Work out the finished part from the listing and answer in its coordinate system (mm). A direction names the side the tool comes from. Give positions to 0.01 mm unless a question says otherwise; leave off trailing zeros. Order: outer loops, then holes, each group sorted by start corner. A loop starts at its lowest first (then second) coordinate and runs counter-clockwise, first axis right, second up. Notation, with made-up numbers: (-18, 53) - (-4, 53) arc R11 ccw to (-4, 63) - close; hole circle Ø10 at (83, 32). An arc over 180 degrees is marked (long way). Put each result on its own line as item: value.
```python
from build123d import *

# Parameters (mm, degrees)
MODEL_R             = 3.6
MODEL_R_2           = 1.7
MODEL_R_3           = 1.500000002
MODEL_W             = 3
MODEL_H             = 9
MODEL_H_2           = 8
BOSS_EXTRUDE1_DEPTH = 3


with BuildPart() as part:
    # Model → Boss-Extrude1 (new body)
    with BuildSketch(Plane.XY):
        with BuildLine():
            Line((39.51904, 20.352307471), (39.51904, 75.773102336))
            Line((39.51904, 75.773102336), (39.51904, 86.677548788))
            ThreePointArc((39.51904, 86.677548788), (33.51909, 92.677598788), (27.51904, 86.677648789))
            Line((27.51904, 86.677648789), (27.51904, 6.677548789))
            ThreePointArc((27.51904, 6.677548789), (33.519039999, 0.677548789), (39.51904, 6.677548789))
            Line((39.51904, 6.677548789), (39.51904, 20.352307471))
        make_face()
        with Locations((33.519039999, 6.677548788)):
            Circle(MODEL_R, mode=Mode.SUBTRACT)
        with Locations((33.519039998, 86.677548787)):
            Circle(MODEL_R_2, mode=Mode.SUBTRACT)
        with Locations((33.519040002, 54.677648787)):
            Circle(MODEL_R_3, mode=Mode.SUBTRACT)
        with Locations((33.51904, 34.177548789)):
            Rectangle(MODEL_W, MODEL_H, mode=Mode.SUBTRACT)
        with Locations((33.51904, 72.677548789)):
            Rectangle(MODEL_W, MODEL_H_2, mode=Mode.SUBTRACT)
        with BuildLine():
            Line((32.61904, 21.677648789), (32.61904, 16.677548789))
            ThreePointArc((32.61904, 16.677548789), (33.51904, 15.777548789), (34.41904, 16.677548789))
            Line((34.41904, 16.677548789), (34.41904, 21.677548786))
            ThreePointArc((34.41904, 21.677548786), (33.519090001, 22.577598787), (32.61904, 21.677648789))
        make_face(mode=Mode.SUBTRACT)
    extrude(amount=BOSS_EXTRUDE1_DEPTH)


solid = part.part
```
(1) Determine the mould class of faces 1 (the face through (33, 47, 0)), 2 (the face through (33.651, 92.676, 1.479)), 3 (the face through (33, 68.678, 1)) for opening direction X: pulls with the +X half, pulls with the -X half, needs draft (parallel to the pull), parting line crosses it, or undercut.
Geometry check:
face 1: needs draft
face 2: parting line crosses it
face 3: undercut
(2) Section A-A, the plane x = 36.25 is taken. Write down the section's boundary in (y, z).
Geometry check:
outline: (1.34, 0) - (4.33, 0) - (4.33, 3) - (1.34, 3) - close; (9.02, 0) - (92.02, 0) - (92.02, 3) - (9.02, 3) - close
(3) A tool of negligible diameter and unlimited length cuts with its end or side. For faces 4 (the face through (39.519, 46, 1)), 5 (the face through (33, 38.678, 1)), from which of +Z, -Z, +X, -X, +Y, -Y can it reach the whole face along a straight path? Write none if from no direction.
Geometry check:
face 4: +Z, -Z, +X, +Y, -Y
face 5: +Z, -Z
(4) Section B-B, the plane z = 1.8 is taken. Write down the section's boundary in (x, y), then the cut area to 3 significant figures.
Geometry check:
outline: (27.52, 6.68) arc R6 ccw to (39.52, 6.68) - (39.52, 86.68) arc R6 ccw to (27.52, 86.68) - close; hole circle Ø7.2 at (33.52, 6.68); hole circle Ø3.4 at (33.52, 86.68); hole (32.02, 29.68) - (35.02, 29.68) - (35.02, 38.68) - (32.02, 38.68) - close; hole circle Ø3 at (33.52, 54.68); hole (32.02, 68.68) - (35.02, 68.68) - (35.02, 76.68) - (32.02, 76.68) - close; hole (32.62, 16.68) arc R0.9 ccw to (34.42, 16.68) - (34.42, 21.68) arc R0.9 ccw to (32.62, 21.68) - close
area: 954 mm²
(5) Straight lines are drawn through the part: line 1 (X direction, y = 35.5, z = 1.9); line 2 (Y direction, x = 32.5, z = 0.9); line 3 (Y direction, x = 34.5, z = 0.4). For each, find the intervals that lie inside material, in ascending order.
Geometry check:
line 1: x = 27.52 to 32.02, 35.02 to 39.52
line 2: y = 0.76 to 3.22, 10.13 to 29.68, 38.68 to 53.58, 55.78 to 68.68, 76.68 to 85.32, 88.04 to 92.59
line 3: y = 0.76 to 3.21, 10.14 to 29.68, 38.68 to 53.54, 55.81 to 68.68, 76.68 to 85.29, 88.07 to 92.6
(6) Given pin 1 (4.5 mm diameter, centred on x = 33.52, y = 6.68, fed in from -Z); pin 2 (5.5 mm diameter, centred on x = 33.52, y = 86.68, fed in from -Z); pin 3 (1.5 mm diameter, centred on x = 34.5, z = 1, fed in from +Y), each flat-ended and moving along its own axis, determine where each tip first touches the part or whether it passes through.
Geometry check:
pin 1: passes through
pin 2: stops at z = 0
pin 3: stops at y = 92.67
